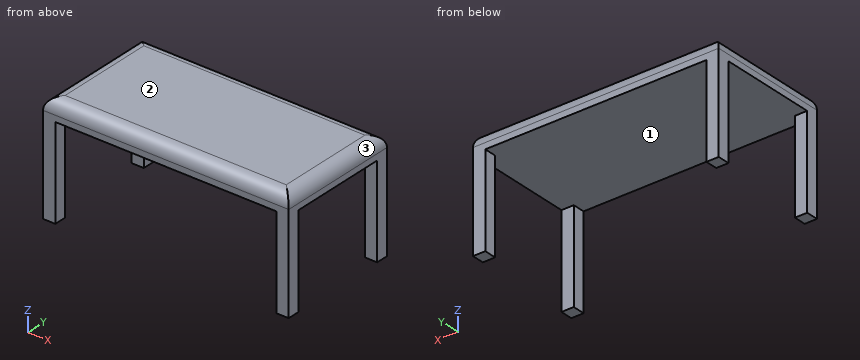
```python
from build123d import *

# Parameters (mm, degrees)
F0_W     = 101.6
F0_H     = 50.8
F1_DEPTH = 7.62
F2_R     = 5.08
F3_W     = 5.08
F3_H     = 5.08
F4_DEPTH = 38.1


with BuildPart() as f1:
    # F0 (on Top) → F1 (new body)
    with BuildSketch(Plane.XY):
        with Locations((-9.186735, -12.039736)):
            Rectangle(F0_W, F0_H)
    extrude(amount=F1_DEPTH)

    # F2
    f2_edges = [f1.edges().sort_by_distance(p)[0] for p in [
        (-9.186735, -37.439736, 7.62),
        (-59.986735, -12.039736, 7.62),
        (-9.186735, 13.360264, 7.62),
        (41.613265, -12.039736, 7.62),
    ]]
    fillet(f2_edges, radius=F2_R)

    # F3 (on face) → F4 (join)
    with BuildSketch(Plane(origin=(0, 0, 0), x_dir=(1, 0, 0), z_dir=(0, 0, -1))):
        with Locations((39.073265, -10.820264)):
            Rectangle(F3_W, F3_H)
        with Locations((39.073265, 34.899736)):
            Rectangle(F3_W, F3_H)
        with Locations((-57.446735, -10.820264)):
            Rectangle(F3_W, F3_H)
        with Locations((-57.446735, 34.899736)):
            Rectangle(F3_W, F3_H)
    extrude(amount=F4_DEPTH)


solid = f1.part
```
Could you check a few things on this model? Use its own coordinates, in mm. Face numbers are marked on the shaded views. Round coordinates to 2 decimals unless told otherwise and drop trailing zeros. Write each loop counter-clockwise with the first axis right and the second up, starting at its lowest first coordinate (ties: lowest second). Pieces come first, ordered by that corner, then holes. Notation, with made-up numbers: M 4,85.5 L 36,85.5 A19 cw 36,111.5 Z; hole C 73,62.25 d1. An arc over 180 degrees is marked long. Answer in a Markdown table with one row per item. Add a question column.
Q1. Imagine slicing it at B-B (x = -24). Please give me the cut outline in (y, z), then the cut area to 3 significant figures.
Q2. If we mould it in two halves opening along X, with no side actions, what happens to the marked faces 1, 2 and 3? For each: +X half, -X half, draft (parallel to the pull), parting line (faces both ways), or undercut.
Q3. Imagine slicing it at A-A (z = -12.5). Please give me the cut outline in (x, y).
Q4. Will this pin go through, and if not, where does the flat tip stop? pin 1 Ø5 at (x, y) = (12.5, -14.5) entering from -Z.
Q5. Imagine slicing it at C-C (y = 7). Please give me the cut outline in (x, z).
Q6. If I drill on line 1 (X direction, y = 10, z = -35); line 2 (Z direction, x = -30, y = -9); line 3 (Z direction, x = 15, y = -34.5), over which ranges is the centre line in solid material (lowest first)? Write a range as from..to.
Values:
| question | item | result |
|---|---|---|
| 1 | outline | M -37.44,0 L 13.36,0 L 13.36,2.54 A5.08 ccw 8.28,7.62 L -32.36,7.62 A5.08 ccw -37.44,2.54 Z |
| 1 | area | 376 mm^2 |
| 2 | face 1 | undercut |
| 2 | face 2 | draft |
| 2 | face 3 | +X half |
| 3 | outline | M -59.99,-37.44 L -54.91,-37.44 L -54.91,-32.36 L -59.99,-32.36 Z; M -59.99,8.28 L -54.91,8.28 L -54.91,13.36 L -59.99,13.36 Z; M 36.53,-37.44 L 41.61,-37.44 L 41.61,-32.36 L 36.53,-32.36 Z; M 36.53,8.28 L 41.61,8.28 L 41.61,13.36 L 36.53,13.36 Z |
| 4 | pin 1 | z = 0 |
| 5 | outline | M -59.99,0 L 41.61,0 L 41.61,2.54 A5.08 ccw 36.53,7.62 L -54.91,7.62 A5.08 ccw -59.99,2.54 Z |
| 6 | line 1 | -59.99..-54.91, 36.53..41.61 |
| 6 | line 2 | 0..7.62 |
| 6 | line 3 | 0..7.15 |
